Print and shaded views of the part. All mm, measured from the part's lowest x, y and z. A direction names the side the tool comes from. Coordinates: 2 decimals unless noted, no trailing zeros. Loops run counter-clockwise (first coordinate to the right, second up) from the corner with the lowest first, then second, coordinate; pieces in that order, holes last. Notation, with made-up numbers: M 88.25,27.5 L 134.25,27.5 A18 cw 134.25,42.5 Z; hole C 34.5,27 d3. An arc over 180 degrees is marked long. One line per question, with ' | ' between items. Start each with the question number.
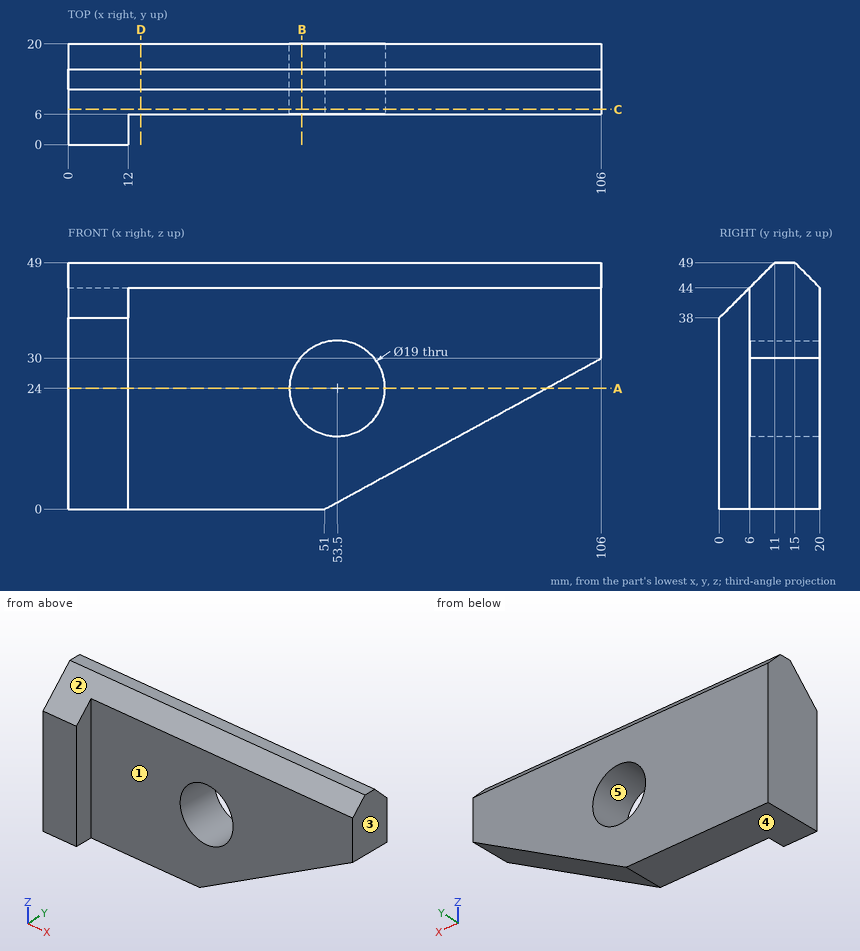
(1) Band-saw the part on B-B on x = 46.5. Write the cut outline in (y, z), then the cut area to 3 significant figures.
(2) Drill centre lines: line 1 (Y direction, x = 26, z = 20); line 2 (X direction, y = 18.25, z = 15.5); line 3 (Z direction, x = 53.5, y = 17.25). Where is each one in solid material? Low to high. Write a range as [from, to].
(3) Band-saw the part on A-A on z = 24. Write the cut outline in (x, y), then the cut area to 3 significant figures.
(4) Two-plate mould, pull along Z, no slides. Class the marked faces 3, 4 and 5: pulls with the +Z half, pulls with the -Z half, needs draft (parallel to the pull), parting line crosses it, or undercut.
(5) Pin check, flat tips, straight feed: P1, Ø6, axis at x = 51, z = 40, coming from the -Y side; P2, Ø1.5, axis at x = 55.5, y = 3.5, coming from the +Z side; P3, Ø3, axis at y = 2, z = 15.5, coming from the +X side. Stop position of each tip, or through.
(6) Band-saw the part on C-C on y = 7. Write the cut outline in (x, z).
(7) Band-saw the part on D-D on x = 14.5. Write the cut outline in (y, z).
(8) 3-axis set-ups, long thin cutter, end or side, ignore diameter. For the marked faces 1 and 2: which of +Z, -Z, +X, -X, +Y, -Y reach the whole face in a straight line?
Computed values:
1) outline: M 6,0 L 20,0 L 20,17.58 L 6,17.58 Z; M 6,30.42 L 20,30.42 L 20,44 L 15,49 L 11,49 L 6,44 Z | area: 481 mm^2
2) line 1: [6, 20] | line 2: [0, 49.26], [57.74, 79.42] | line 3: [1.36, 14.5], [33.5, 46.75]
3) outline: M 0,0 L 12,0 L 12,6 L 44,6 L 44,20 L 0,20 Z; M 63,6 L 95,6 L 95,20 L 63,20 Z | area: 1,140 mm^2
4) face 3: needs draft | face 4: pulls with the -Z half | face 5: undercut
5) P1: y = 6 | P2: through | P3: x = 12
6) outline: M 0,0 L 51,0 L 106,30 L 106,45 L 0,45 Z; hole C 53.5,24 d19
7) outline: M 6,0 L 20,0 L 20,44 L 15,49 L 11,49 L 6,44 Z
8) face 1: +Z, -Z, +X, -Y | face 2: +Z, +X, -X, -Y
